The model under review builds one solid part; all positions refer to its coordinate system, in mm. Face numbers are marked on the shaded views. A direction names the side the tool comes from. Round coordinates to 2 decimals unless told otherwise and drop trailing zeros. Write each loop counter-clockwise with the first axis right and the second up, starting at its lowest first coordinate (ties: lowest second). Pieces come first, ordered by that corner, then holes. Notation, with made-up numbers: (63.25, -26) - (97.25, -26) arc R18 ccw to (97.25, 2) - close; hole circle Ø5 at (-19.75, 38). An arc over 180 degrees is marked (long way). Return JSON: item names as keys, results as strings.
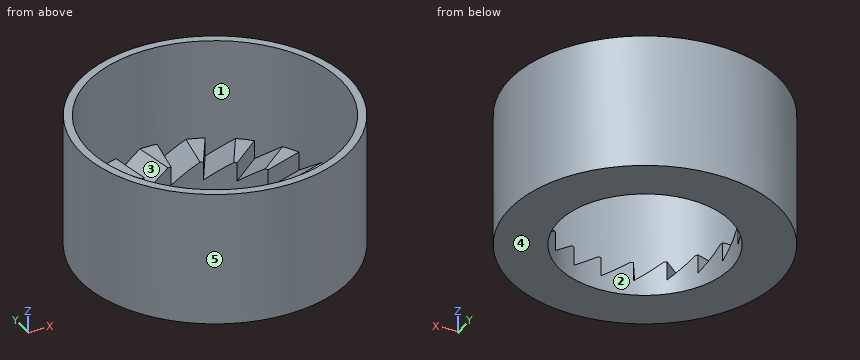
from build123d import *

# Parameters (mm, degrees)
F0_R            = 20
F1_DEPTH        = 20
F2_R            = 18.8
F3_DEPTH        = 15
F4_R            = 12.8
F5_DEPTH        = 25
F7_END_RADIUS   = 18.8
F7_REACH        = 24.884098355
F7_COPIES_COUNT = 18


# Not quite as in the source:
# - a pattern or mirror of a feature is missing from the dataset's text; its kind, count and spacing are read off the source's solid


with BuildPart() as f1:
    # F0 (on Top) → F1 (new body)
    with BuildSketch(Plane.XY):
        Circle(F0_R)
    extrude(amount=F1_DEPTH)

    # F2 (on face) → F3 (cut)
    with BuildSketch(Plane.XY.offset(20)):
        Circle(F2_R)
    extrude(amount=-F3_DEPTH, mode=Mode.SUBTRACT)

    # F4 (on face) → F5 (cut)
    with BuildSketch(Plane.XY.offset(5)):
        Circle(F4_R)
    extrude(amount=-F5_DEPTH, mode=Mode.SUBTRACT)

    f7_end = (Plane.XY.offset(12.5) * Cylinder(F7_END_RADIUS, 169.7681967101, mode=Mode.PRIVATE)).faces().sort_by_distance((-18.8, 0, 12.5))[0]
    # F6 (on Right) → F7 (cut, up to the whole of a round face its end follows)
    with BuildSketch(Plane.YZ):
        Polygon((-2, 5), (-2, 2.1991698472), (0, 3.5995849236), (2, 5), align=None)
    f7_long = extrude(amount=-F7_REACH, mode=Mode.PRIVATE)
    f7 = split(f7_long, bisect_by=f7_end, keep=Keep.BOTTOM, mode=Mode.PRIVATE)
    add(f7, mode=Mode.SUBTRACT)

    # F7_copies: F7 ×18 about axis
    f7_copies_axis = Axis((0, 0, 0), (0, 0, 1))
    for i in range(1, F7_COPIES_COUNT):
        add(f7.rotate(f7_copies_axis, i * 360 / F7_COPIES_COUNT), mode=Mode.SUBTRACT)


solid = f1.part
(1) Mouldability with a two-part tool opening along X and no side actions: class the marked faces 3, 4 and 5 as released by +X, released by -X, zero draft, split by the parting line, or undercut.
Filled in:
{"face 3": "undercut", "face 4": "zero draft", "face 5": "split by the parting line"}
(2) Add section A-A (y = 3.5). Write out the cut boundary in (x, z), plus the area to 3 significant figures.
Filled in:
{"outline": "(-19.69, 0) - (-12.31, 0) - (-12.31, 2.95) - (-15.46, 2.2) - (-15.46, 5) - (-18.47, 5) - (-18.47, 20) - (-19.69, 20) - close; (12.31, 0) - (19.69, 0) - (19.69, 20) - (18.47, 20) - (18.47, 5) - (15.46, 5) - (12.31, 4.25) - close", "area": "102 mm2"}
(3) For the marked faces 1 and 2, list the 3-axis set-ups (+Z, -Z, +X, -X, +Y, -Y) from which the entire face can be reached by the end or side of a thin tool; tool diameter is ignored.
Filled in:
{"face 1": "+Z", "face 2": "+Z, -Z"}
(4) Wall thickness on line 1 (Y direction, x = 0, z = 1.35); line 2 (Y direction, x = 0, z = 13.75); line 3 (X direction, y = 9, z = 1): over which ranges is each line inside the solid? List them lowest first.
Filled in:
{"line 1": "y = -20 to -12.8, 12.8 to 20", "line 2": "y = -20 to -18.8, 18.8 to 20", "line 3": "x = -17.86 to -9.1, 9.1 to 17.86"}
(5) Add section D-D (x = 14). Write out the cut boundary in (y, z).
Filled in:
{"outline": "(-14.28, 0) - (14.28, 0) - (14.28, 20) - (12.55, 20) - (12.55, 3.17) - (9.14, 5) - (7.22, 5) - (7.22, 2.2) - (2.97, 5) - (2, 5) - (2, 2.2) - (-2, 5) - (-2.97, 5) - (-2.97, 2.2) - (-7.22, 5) - (-9.14, 5) - (-9.14, 2.2) - (-12.55, 4.03) - (-12.55, 20) - (-14.28, 20) - close"}
(6) Clearance check with flat-ended pins moving along their axes: pin 1 Ø6 at (y, z) = (14.5, 3.5) entering from +X; pin 2 Ø0.8 at (x, y) = (-15.5, -3.5) entering from +Z; pin 3 Ø10 at (y, z) = (-11, 12) entering from -X. State where each tip first meets the part, or that it passes through.
Filled in:
{"pin 1": "stops at x = 16.36", "pin 2": "stops at z = 5", "pin 3": "stops at x = -19.08"}
(7) Add section C-C (z = 12). Write out the cut boundary in (x, y).
Filled in:
{"outline": "circle Ø40 at (0, 0); hole circle Ø37.6 at (0, 0)"}
(8) Add section B-B (x = -6.5). Write out the cut boundary in (y, z).
Filled in:
{"outline": "(-18.91, 0) - (-11.03, 0) - (-11.03, 3.68) - (-15.26, 2.2) - (-15.26, 5) - (-17.64, 5) - (-17.64, 20) - (-18.91, 20) - close; (11.03, 0) - (18.91, 0) - (18.91, 20) - (17.64, 20) - (17.64, 5) - (15.26, 5) - (11.03, 3.52) - close"}
